Read the model definition and answer for the solid it produces. Units are mm, in the model's axes. A direction names the side the tool comes from. Give positions to 0.01 mm unless a question says otherwise; leave off trailing zeros. Order: outer loops, then holes, each group sorted by start corner. A loop starts at its lowest first (then second) coordinate and runs counter-clockwise, first axis right, second up.
Autodesk Fusion 360 part; units mm, degrees
sketch "Boceto1" plane through (0, 0, 0) normal (0, 1, 0) x (1, 0, 0)
  line L0 (0, 0) -> (97.6, 0)
  line L1 (97.6, 0) -> (97.6, 26.186)
  line L2 (97.6, 26.186) -> (0, 26.186)
  line L3 (0, 26.186) -> (0, 0)
  dimension "d1" = 97.6
  dimension "d2" = 26.186
extrude "Extruir1" add sketch "Boceto1" along normal blind 2
sketch "Boceto2" plane through (0, 2, 0) normal (0, 1, 0) x (-1, 0, 0)
  line L0 (0, -26.186) -> (0, 0)
  line L1 (0, 0) -> (-97.6, 0)
  line L2 (-97.6, 0) -> (-97.6, -26.186)
  line L3 (-97.6, -26.186) -> (0, -26.186)
  line L4 (-97.6, -26.186) -> (-97.6, -13.093)
  line L5 (-97.6, -13.093) -> (-104.1, -13.093)
  circle A0 centre (-104.1, -13.093) radius 1.6
  line L6 (-97.6, -26.186) -> (-97.6, -21.186)
  line L7 (-97.6, -21.186) -> (-110.6, -21.186)
  line L8 (-110.6, -21.186) -> (-110.6, -5)
  line L9 (-110.6, -5) -> (-97.6, -5)
  line L10 (-97.6, -5) -> (-97.6, -21.186)
  dimension "d5" = 13.093
  dimension "d6" = 6.5
  dimension "d7" = 3.2
  dimension "d8" = 5
  dimension "d9" = 13
  dimension "d10" = 16.186
extrude "Extruir2" add sketch "Boceto2" against normal blind 2 contours L2 L4 L7 L8 L9 L10
sketch "Boceto3" plane through (0, 2, 0) normal (0, 1, 0) x (-1, 0, 0)
  circle A0 centre (-104.1, -13.093) radius 1.6
  line L0 (0, -26.186) -> (0, 0)
  line L1 (0, 0) -> (-97.6, 0)
  line L2 (-97.6, 0) -> (-97.6, -5)
  line L3 (-97.6, -5) -> (-110.6, -5)
  line L4 (-110.6, -5) -> (-110.6, -21.186)
  line L5 (-110.6, -21.186) -> (-97.6, -21.186)
  line L6 (-97.6, -21.186) -> (-97.6, -26.186)
  line L7 (-97.6, -26.186) -> (0, -26.186)
  line L8 (0, -26.186) -> (0, -21.186)
  line L9 (0, -21.186) -> (13, -21.186)
  line L10 (13, -21.186) -> (13, -5)
  line L11 (13, -5) -> (0, -5)
  line L12 (0, -5) -> (0, -21.186)
  line L13 (0, -26.186) -> (0, -13.093)
  line L14 (0, -13.093) -> (6.5, -13.093)
  circle A1 centre (6.5, -13.093) radius 1.6
  dimension "d13" = 5
  dimension "d14" = 13
  dimension "d15" = 16.186
  dimension "d16" = 13.093
  dimension "d17" = 6.5
  dimension "d18" = 3.2
extrude "Extruir3" add sketch "Boceto3" against normal blind 2 contours L0 L9 L10 L11 L12 L13
sketch "Boceto4" plane through (0, 2, 0) normal (0, 1, 0) x (-1, 0, 0)
  circle A0 centre (6.5, -13.093) radius 1.6
  circle A1 centre (-104.1, -13.093) radius 1.6
  line L0 (0, -26.186) -> (0, -21.186)
  line L1 (0, -21.186) -> (13, -21.186)
  line L2 (13, -21.186) -> (13, -5)
  line L3 (13, -5) -> (0, -5)
  line L4 (0, -5) -> (0, 0)
  line L5 (0, 0) -> (-97.6, 0)
  line L6 (-97.6, 0) -> (-97.6, -5)
  line L7 (-97.6, -5) -> (-110.6, -5)
  line L8 (-110.6, -5) -> (-110.6, -21.186)
  line L9 (-110.6, -21.186) -> (-97.6, -21.186)
  line L10 (-97.6, -21.186) -> (-97.6, -26.186)
  line L11 (-97.6, -26.186) -> (0, -26.186)
  line L12 (-96.6, -6) -> (-109.6, -6)
  line L13 (-109.6, -6) -> (-109.6, -20.186)
  line L14 (-109.6, -20.186) -> (-96.6, -20.186)
  line L15 (-96.6, -20.186) -> (-96.6, -25.186)
  line L16 (-96.6, -25.186) -> (-1, -25.186)
  line L17 (-1, -25.186) -> (-1, -20.186)
  line L18 (-1, -20.186) -> (12, -20.186)
  line L19 (12, -20.186) -> (12, -6)
  line L20 (12, -6) -> (-1, -6)
  line L21 (-1, -6) -> (-1, -1)
  line L22 (-1, -1) -> (-96.6, -1)
  line L23 (-96.6, -1) -> (-96.6, -6)
  dimension "d21" = -1
extrude "Extruir4" cut sketch "Boceto4" against normal blind 2 contours L0 L1 L2 L3 L4 L5 L6 L7 L8 L9 L10 L11
equation "d5 = 26.186 * 0.5 mm"
equation "d6 = ( 13 * 0.5 ) * 1 mm"
equation "d10 = 21.186 mm - 5 mm"
equation "d15 = 21.186 mm - 5 mm"
equation "d16 = 26.186 * 0.5 mm"
equation "d17 = 13.000 * 0.5 mm"
1) The part is cut by section A-A on x = -6.5. Determine the outline of the cut face in (y, z), and give its area (3 significant figures).
Final values:
outline: (0, -20.19) - (2, -20.19) - (2, -14.69) - (0, -14.69) - close; (0, -11.49) - (2, -11.49) - (2, -6) - (0, -6) - close
area: 22.0 mm2
2) For a pull along Z with two mould halves and no side action, classify faces 5 (the face through (49, 1, -25.186)), 6 (the face through (-7.24, 1.01, -14.51)), 7 (the face through (96.6, 1, -23)), 8 (the face through (48, 1, -1)) as released by +Z, released by -Z, zero draft, split by the parting line, or undercut.
Final values:
face 5: released by -Z
face 6: undercut
face 7: zero draft
face 8: released by +Z
3) Consider L1, parallel to Z at x = 104.1, y = 1.5; L2, parallel to X at y = 1.5, z = -13.5; L3, parallel to X at y = 0.45, z = -22.25. Determine where each line is inside the solid, lowest interval first.
Final values:
L1: z = -20.19 to -14.69, -11.49 to -6
L2: x = -12 to -8.05, -4.95 to 102.55, 105.65 to 109.6
L3: x = 1 to 96.6
4) A tool of negligible diameter and unlimited length cuts with its end or side. For faces 1 (the face through (-6, 1, -6)), 2 (the face through (1, 1, -23)), 3 (the face through (103, 1, -20.186)), 4 (the face through (96.6, 1, -3)), from which of +Z, -Z, +X, -X, +Y, -Y can it reach the whole face along a straight path? Write none if from no direction.
Final values:
face 1: +Z, -X, +Y, -Y
face 2: -Z, -X, +Y, -Y
face 3: -Z, +X, +Y, -Y
face 4: +Z, +X, +Y, -Y
5) The part is cut by section D-D on x = 98.5. Determine the outline of the cut face in (y, z).
Final values:
outline: (0, -20.19) - (2, -20.19) - (2, -6) - (0, -6) - close
6) The part is cut by section B-B on y = 0.5. Determine the outline of the cut face in (x, z).
Final values:
outline: (-12, -20.19) - (1, -20.19) - (1, -25.19) - (96.6, -25.19) - (96.6, -20.19) - (109.6, -20.19) - (109.6, -6) - (96.6, -6) - (96.6, -1) - (1, -1) - (1, -6) - (-12, -6) - close; hole circle Ø3.2 at (-6.5, -13.09); hole circle Ø3.2 at (104.1, -13.09)
7) Given pin 1 (0.6 mm diameter, centred on x = -5, y = 0.5, fed in from +Z); pin 2 (1 mm diameter, centred on y = 1, z = -4.5, fed in from +X); pin 3 (1.9 mm diameter, centred on x = 104.1, z = -13.093, fed in from +Y); pin 4 (0.6 mm diameter, centred on y = 1, z = -24, fed in from -X), each flat-ended and moving along its own axis, determine where each tip first touches the part or whether it passes through.
Final values:
pin 1: stops at z = -6
pin 2: stops at x = 96.6
pin 3: passes through
pin 4: stops at x = 1
8) The part is cut by section C-C on z = -5. Determine the outline of the cut face in (x, y).
Final values:
outline: (1, 0) - (96.6, 0) - (96.6, 2) - (1, 2) - close
